from build123d import *

# Parameters (mm, degrees)
F0_W         = 38
F0_H         = 45
F1_DEPTH     = 35
F2_W         = 13
F2_H         = 25
F2_R         = 1.25
F3_DEPTH     = 16
F4_T1_DEPTH  = 32
F4_T3_DEPTH  = 39
F4_T5_DEPTH  = 29
F4_S9_W      = 3
F4_S9_H      = 3
F4_T10_DEPTH = 3
F4_S15_W     = 3
F4_S15_H     = 3
F4_T16_DEPTH = 3
F4_S21_W     = 3
F4_S21_H     = 3
F4_T22_DEPTH = 3
F4_S27_W     = 3
F4_S27_H     = 3
F4_T28_DEPTH = 3
F4_S33_W     = 3
F4_S33_H     = 3
F4_T34_DEPTH = 3
F4_S39_W     = 3
F4_S39_H     = 3
F4_T40_DEPTH = 3
F4_S45_W     = 3
F4_S45_H     = 3
F4_T46_DEPTH = 3
F4_S51_W     = 3
F4_S51_H     = 3
F4_T52_DEPTH = 3
F5_R         = 1.25
F6_DEPTH     = 7


# Not quite as in the source:
# - a fillet or chamfer that OpenCascade refuses, or shapes differently, is made with other operations: its cross-section is extruded or revolved along the edge and cut away or added


with BuildPart() as f1:
    # F0 (on Top) → F1 (new body)
    with BuildSketch(Plane.XY):
        with Locations((4.8651863657, 11.567664966)):
            Rectangle(F0_W, F0_H)
    extrude(amount=F1_DEPTH)

    # F2 (on face) → F3 (cut)
    with BuildSketch(Plane(origin=(-14.1348136343, 0, 0), x_dir=(0, -1, 0), z_dir=(-1, 0, 0))):
        with Locations((-25.067664966, 17.5)):
            Rectangle(F2_W, F2_H)
        with Locations((1.932335034, 17.5)):
            Rectangle(F2_W, F2_H)
        with Locations((1.932335034, 32.25)):
            Circle(F2_R)
        with Locations((1.932335034, 2.75)):
            Circle(F2_R)
        with Locations((-25.067664966, 32.25)):
            Circle(F2_R)
        with Locations((-25.067664966, 2.75)):
            Circle(F2_R)
    extrude(amount=-F3_DEPTH, mode=Mode.SUBTRACT)

    # F4: fillet of radius 3 on 12 edges, made by hand

    # F4_s2 → F4_t1 (cut)
    with BuildSketch(Plane.YZ.offset(-11.1348136343)):
        with BuildLine():
            ThreePointArc((34.067664966, 3), (33.1889853095, 0.8786796564), (31.067664966, 0))
            Line((31.067664966, 0), (34.067664966, 0))
            Line((34.067664966, 0), (34.067664966, 3))
        make_face()
        with BuildLine():
            ThreePointArc((34.067664966, 32), (33.1889853095, 34.1213203436), (31.067664966, 35))
            Line((31.067664966, 35), (34.067664966, 35))
            Line((34.067664966, 35), (34.067664966, 32))
        make_face()
        with BuildLine():
            ThreePointArc((-7.932335034, 0), (-10.0536553776, 0.8786796564), (-10.932335034, 3))
            Line((-10.932335034, 3), (-10.932335034, 0))
            Line((-10.932335034, 0), (-7.932335034, 0))
        make_face()
        with BuildLine():
            ThreePointArc((-7.932335034, 35), (-10.0536553776, 34.1213203436), (-10.932335034, 32))
            Line((-10.932335034, 32), (-10.932335034, 35))
            Line((-10.932335034, 35), (-7.932335034, 35))
        make_face()
    extrude(amount=F4_T1_DEPTH, mode=Mode.SUBTRACT)

    # F4_s4 → F4_t3 (cut)
    with BuildSketch(Plane.XZ.offset(-31.067664966)):
        with BuildLine():
            ThreePointArc((20.8651863657, 35), (22.9865067092, 34.1213203436), (23.8651863657, 32))
            Line((23.8651863657, 32), (23.8651863657, 35))
            Line((23.8651863657, 35), (20.8651863657, 35))
        make_face()
        with BuildLine():
            ThreePointArc((20.8651863657, 0), (22.9865067092, 0.8786796564), (23.8651863657, 3))
            Line((23.8651863657, 3), (23.8651863657, 0))
            Line((23.8651863657, 0), (20.8651863657, 0))
        make_face()
        with BuildLine():
            ThreePointArc((-14.1348136343, 32), (-13.2561339779, 34.1213203436), (-11.1348136343, 35))
            Line((-11.1348136343, 35), (-14.1348136343, 35))
            Line((-14.1348136343, 35), (-14.1348136343, 32))
        make_face()
        with BuildLine():
            ThreePointArc((-14.1348136343, 3), (-13.2561339779, 0.8786796564), (-11.1348136343, 0))
            Line((-11.1348136343, 0), (-14.1348136343, 0))
            Line((-14.1348136343, 0), (-14.1348136343, 3))
        make_face()
    extrude(amount=F4_T3_DEPTH, mode=Mode.SUBTRACT)

    # F4_s6 → F4_t5 (cut)
    with BuildSketch(Plane.XY.offset(3)):
        with BuildLine():
            ThreePointArc((20.8651863657, 34.067664966), (22.9865067092, 33.1889853095), (23.8651863657, 31.067664966))
            Line((23.8651863657, 31.067664966), (23.8651863657, 34.067664966))
            Line((23.8651863657, 34.067664966), (20.8651863657, 34.067664966))
        make_face()
        with BuildLine():
            ThreePointArc((20.8651863657, -10.932335034), (22.9865067092, -10.0536553776), (23.8651863657, -7.932335034))
            Line((23.8651863657, -7.932335034), (23.8651863657, -10.932335034))
            Line((23.8651863657, -10.932335034), (20.8651863657, -10.932335034))
        make_face()
        with BuildLine():
            ThreePointArc((-14.1348136343, 31.067664966), (-13.2561339779, 33.1889853095), (-11.1348136343, 34.067664966))
            Line((-11.1348136343, 34.067664966), (-14.1348136343, 34.067664966))
            Line((-14.1348136343, 34.067664966), (-14.1348136343, 31.067664966))
        make_face()
        with BuildLine():
            ThreePointArc((-14.1348136343, -7.932335034), (-13.2561339779, -10.0536553776), (-11.1348136343, -10.932335034))
            Line((-11.1348136343, -10.932335034), (-14.1348136343, -10.932335034))
            Line((-14.1348136343, -10.932335034), (-14.1348136343, -7.932335034))
        make_face()
    extrude(amount=F4_T5_DEPTH, mode=Mode.SUBTRACT)


with BuildPart() as f4_tool8:
    # F4_s9 → F4_t10 (new body)
    with BuildSketch(Plane.XZ.offset(-31.067664966)):
        with Locations((22.3651863657, 1.5)):
            Rectangle(F4_S9_W, F4_S9_H)
    extrude(amount=-F4_T10_DEPTH)

    # F4_s11 → F4_t12 (revolve, cut)
    with BuildSketch(Plane(origin=(20.8651863657, 31.067664966, 3), x_dir=(-0.7071067812, 0, 0.7071067812), z_dir=(-0.7071067812, 0, -0.7071067812))):
        with BuildLine():
            ThreePointArc((0, -3), (3, 0), (0, 3))
            Line((0, 3), (0, -3))
        make_face()
    revolve(axis=Axis((20.8651863657, 31.067664966, 3), (0, 1, 0)), mode=Mode.SUBTRACT)


with BuildPart() as f1_1:
    add(f1.part)

    # F4_t7: cut F4_tool8
    add(f4_tool8.part, mode=Mode.SUBTRACT)


with BuildPart() as f4_tool14:
    # F4_s15 → F4_t16 (new body)
    with BuildSketch(Plane.YZ.offset(-11.1348136343)):
        with Locations((32.567664966, 1.5)):
            Rectangle(F4_S15_W, F4_S15_H)
    extrude(amount=-F4_T16_DEPTH)

    # F4_s17 → F4_t18 (revolve, cut)
    with BuildSketch(Plane(origin=(-11.1348136343, 31.067664966, 3), x_dir=(0, -0.7071067812, 0.7071067812), z_dir=(0, -0.7071067812, -0.7071067812))):
        with BuildLine():
            ThreePointArc((0, -3), (3, 0), (0, 3))
            Line((0, 3), (0, -3))
        make_face()
    revolve(axis=Axis((-11.1348136343, 31.067664966, 3), (-1, 0, 0)), mode=Mode.SUBTRACT)


with BuildPart() as f1_2:
    add(f1_1.part)

    # F4_t13: cut F4_tool14
    add(f4_tool14.part, mode=Mode.SUBTRACT)


with BuildPart() as f4_tool20:
    # F4_s21 → F4_t22 (new body)
    with BuildSketch(Plane.XZ.offset(-31.067664966)):
        with Locations((22.3651863657, 33.5)):
            Rectangle(F4_S21_W, F4_S21_H)
    extrude(amount=-F4_T22_DEPTH)

    # F4_s23 → F4_t24 (revolve, cut)
    with BuildSketch(Plane(origin=(20.8651863657, 31.067664966, 32), x_dir=(-0.7071067812, 0, -0.7071067812), z_dir=(0.7071067812, 0, -0.7071067812))):
        with BuildLine():
            ThreePointArc((0, -3), (3, 0), (0, 3))
            Line((0, 3), (0, -3))
        make_face()
    revolve(axis=Axis((20.8651863657, 31.067664966, 32), (0, 1, 0)), mode=Mode.SUBTRACT)


with BuildPart() as f1_3:
    add(f1_2.part)

    # F4_t19: cut F4_tool20
    add(f4_tool20.part, mode=Mode.SUBTRACT)


with BuildPart() as f4_tool26:
    # F4_s27 → F4_t28 (new body)
    with BuildSketch(Plane.YZ.offset(-11.1348136343)):
        with Locations((32.567664966, 33.5)):
            Rectangle(F4_S27_W, F4_S27_H)
    extrude(amount=-F4_T28_DEPTH)

    # F4_s29 → F4_t30 (revolve, cut)
    with BuildSketch(Plane(origin=(-11.1348136343, 31.067664966, 32), x_dir=(0, -0.7071067812, -0.7071067812), z_dir=(0, 0.7071067812, -0.7071067812))):
        with BuildLine():
            ThreePointArc((0, -3), (3, 0), (0, 3))
            Line((0, 3), (0, -3))
        make_face()
    revolve(axis=Axis((-11.1348136343, 31.067664966, 32), (-1, 0, 0)), mode=Mode.SUBTRACT)


with BuildPart() as f1_4:
    add(f1_3.part)

    # F4_t25: cut F4_tool26
    add(f4_tool26.part, mode=Mode.SUBTRACT)


with BuildPart() as f4_tool32:
    # F4_s33 → F4_t34 (new body)
    with BuildSketch(Plane.YZ.offset(-11.1348136343)):
        with Locations((-9.432335034, 1.5)):
            Rectangle(F4_S33_W, F4_S33_H)
    extrude(amount=-F4_T34_DEPTH)

    # F4_s35 → F4_t36 (revolve, cut)
    with BuildSketch(Plane(origin=(-11.1348136343, -7.932335034, 3), x_dir=(0, 0.7071067812, 0.7071067812), z_dir=(0, -0.7071067812, 0.7071067812))):
        with BuildLine():
            ThreePointArc((0, -3), (3, 0), (0, 3))
            Line((0, 3), (0, -3))
        make_face()
    revolve(axis=Axis((-11.1348136343, -7.932335034, 3), (-1, 0, 0)), mode=Mode.SUBTRACT)


with BuildPart() as f1_5:
    add(f1_4.part)

    # F4_t31: cut F4_tool32
    add(f4_tool32.part, mode=Mode.SUBTRACT)


with BuildPart() as f4_tool38:
    # F4_s39 → F4_t40 (new body)
    with BuildSketch(Plane.YZ.offset(20.8651863657)):
        with Locations((-9.432335034, 1.5)):
            Rectangle(F4_S39_W, F4_S39_H)
    extrude(amount=F4_T40_DEPTH)

    # F4_s41 → F4_t42 (revolve, cut)
    with BuildSketch(Plane(origin=(20.8651863657, -7.932335034, 3), x_dir=(0, 0.7071067812, 0.7071067812), z_dir=(0, 0.7071067812, -0.7071067812))):
        with BuildLine():
            ThreePointArc((0, -3), (3, 0), (0, 3))
            Line((0, 3), (0, -3))
        make_face()
    revolve(axis=Axis((20.8651863657, -7.932335034, 3), (1, 0, 0)), mode=Mode.SUBTRACT)


with BuildPart() as f1_6:
    add(f1_5.part)

    # F4_t37: cut F4_tool38
    add(f4_tool38.part, mode=Mode.SUBTRACT)


with BuildPart() as f4_tool44:
    # F4_s45 → F4_t46 (new body)
    with BuildSketch(Plane.YZ.offset(-11.1348136343)):
        with Locations((-9.432335034, 33.5)):
            Rectangle(F4_S45_W, F4_S45_H)
    extrude(amount=-F4_T46_DEPTH)

    # F4_s47 → F4_t48 (revolve, cut)
    with BuildSketch(Plane(origin=(-11.1348136343, -7.932335034, 32), x_dir=(0, 0.7071067812, -0.7071067812), z_dir=(0, 0.7071067812, 0.7071067812))):
        with BuildLine():
            ThreePointArc((0, -3), (3, 0), (0, 3))
            Line((0, 3), (0, -3))
        make_face()
    revolve(axis=Axis((-11.1348136343, -7.932335034, 32), (-1, 0, 0)), mode=Mode.SUBTRACT)


with BuildPart() as f1_7:
    add(f1_6.part)

    # F4_t43: cut F4_tool44
    add(f4_tool44.part, mode=Mode.SUBTRACT)


with BuildPart() as f4_tool50:
    # F4_s51 → F4_t52 (new body)
    with BuildSketch(Plane.YZ.offset(20.8651863657)):
        with Locations((-9.432335034, 33.5)):
            Rectangle(F4_S51_W, F4_S51_H)
    extrude(amount=F4_T52_DEPTH)

    # F4_s53 → F4_t54 (revolve, cut)
    with BuildSketch(Plane(origin=(20.8651863657, -7.932335034, 32), x_dir=(0, 0.7071067812, -0.7071067812), z_dir=(0, -0.7071067812, -0.7071067812))):
        with BuildLine():
            ThreePointArc((0, -3), (3, 0), (0, 3))
            Line((0, 3), (0, -3))
        make_face()
    revolve(axis=Axis((20.8651863657, -7.932335034, 32), (1, 0, 0)), mode=Mode.SUBTRACT)


with BuildPart() as f1_8:
    add(f1_7.part)

    # F4_t49: cut F4_tool50
    add(f4_tool50.part, mode=Mode.SUBTRACT)

    # F5 (on face) → F6 (cut)
    with BuildSketch(Plane.YZ.offset(23.8651863657)):
        with Locations((-1.932335034, 23.75)):
            Circle(F5_R)
        with Locations((-2.2813694086, 11.25)):
            Circle(F5_R)
        with Locations((25.067664966, 23.75)):
            Circle(F5_R)
        with Locations((25.067664966, 11.25)):
            Circle(F5_R)
    extrude(amount=-F6_DEPTH, mode=Mode.SUBTRACT)


solid = f1_8.part
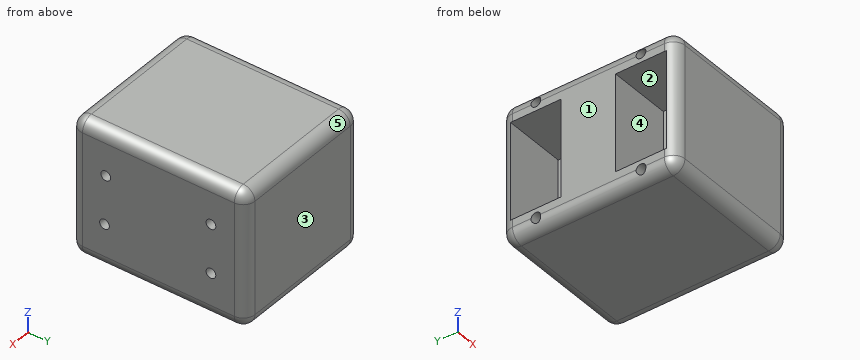
The listing builds one solid part. Answer for the finished solid, in the listing's coordinates (mm). Face numbers are marked on the shaded views. A direction names the side the tool comes from. Round coordinates to 2 decimals unless told otherwise and drop trailing zeros. Write each loop counter-clockwise with the first axis right and the second up, starting at its lowest first coordinate (ties: lowest second). Pieces come first, ordered by that corner, then holes. Notation, with made-up numbers: M -18,-16 L 30,-16 A30 ccw 30,9 Z; hole C 52.5,-14.75 d1. An arc over 180 degrees is marked long. Write each question's results on one line, items separated by ' | '. Start each with the question number.
(1) Determine the mould class of the marked faces 1, 2 and 3 for opening direction Y: +Y half, -Y half, draft (parallel to the pull), parting line (faces both ways), or undercut.
(2) For the marked faces 4 and 5, determine the directions among +Z, -Z, +X, -X, +Y, -Y from which every point of the face is accessible in a straight line to the end or side of a thin tool.
(3) Find the intervals of material crossed by line 1 (Y direction, x = -3, z = 27); line 2 (Y direction, x = -1, z = 32); line 3 (X direction, y = 1, z = 29), in increasing order.
(4) The part is cut by section A-A, the plane x = -6. Write down the section's boundary in (y, z), and give its area (3 significant figures).
(5) The part is cut by section C-C, the plane y = 22. Write down the section's boundary in (x, z), and give its area (3 significant figures).
(6) Each of these flat-tipped pins is pushed along its axis until it touches: P1, Ø2, axis at y = -2.5, z = 11.5, coming from the +X side; P2, Ø2, axis at y = 20, z = 11, coming from the -X side. Where does it stop, or does it pass through?
(7) The part is cut by section D-D, the plane x = -12. Write down the section's boundary in (y, z), and give its area (3 significant figures).
(8) The part is cut by section B-B, the plane z = 11.25. Write down the section's boundary in (x, y).
Worked answers:
1) face 1: draft | face 2: undercut | face 3: +Y half
2) face 4: -X | face 5: +Z, +X, -X, +Y
3) line 1: y = -10.93 to -8.43, 4.57 to 18.57, 31.57 to 34.07 | line 2: y = -10.93 to -3.16, -0.71 to 23.84, 26.29 to 34.07 | line 3: x = 1.87 to 23.87
4) outline: M -10.93,3 A3 ccw -7.93,0 L 31.07,0 A3 ccw 34.07,3 L 34.07,32 A3 ccw 31.07,35 L -7.93,35 A3 ccw -10.93,32 Z; hole M -8.43,5 L 4.57,5 L 4.57,30 L -8.43,30 Z; hole C -1.93,2.75 d2.5; hole C -1.93,32.25 d2.5; hole M 18.57,5 L 31.57,5 L 31.57,30 L 18.57,30 Z; hole C 25.07,2.75 d2.5; hole C 25.07,32.25 d2.5 | area: 898 mm²
5) outline: M -14.13,3 A3 ccw -11.13,0 L 20.87,0 A3 ccw 23.87,3 L 23.87,32 A3 ccw 20.87,35 L -11.13,35 A3 ccw -14.13,32 L -14.13,30 L 1.87,30 L 1.87,5 L -14.13,5 Z | area: 922 mm²
6) P1: stops at x = 23.87 | P2: stops at x = 1.87
7) outline: M -10.8,3 A2.87 ccw -7.93,0.13 L 31.07,0.13 A2.87 ccw 33.94,3 L 33.94,32 A2.87 ccw 31.07,34.87 L -7.93,34.87 A2.87 ccw -10.8,32 Z; hole M -8.43,5 L 4.57,5 L 4.57,30 L -8.43,30 Z; hole C -1.93,2.75 d2.5; hole C -1.93,32.25 d2.5; hole M 18.57,5 L 31.57,5 L 31.57,30 L 18.57,30 Z; hole C 25.07,2.75 d2.5; hole C 25.07,32.25 d2.5 | area: 878 mm²
8) outline: M -14.13,4.57 L 1.87,4.57 L 1.87,-8.43 L -14.09,-8.43 A3 ccw -11.13,-10.93 L 20.87,-10.93 A3 ccw 23.87,-7.93 L 23.87,-3.53 L 16.87,-3.53 L 16.87,-1.03 L 23.87,-1.03 L 23.87,23.82 L 16.87,23.82 L 16.87,26.32 L 23.87,26.32 L 23.87,31.07 A3 ccw 20.87,34.07 L -11.13,34.07 A3 ccw -14.09,31.57 L 1.87,31.57 L 1.87,18.57 L -14.13,18.57 Z
